```python
from build123d import *

# Parameters (mm, degrees)
F2_W           = 40
F2_H           = 40
F3_DEPTH       = 500
F4_R           = 3
F5_T           = -2
F7_DEPTH       = 40.001
F9_D           = 3.5
F9_CSINK_D     = 6
F9_CSINK_ANGLE = 90


with BuildPart() as f3:
    # F2 (on Front) → F3 (new body, symmetric)
    with BuildSketch(Plane.XZ):
        Rectangle(F2_W, F2_H)
    extrude(amount=F3_DEPTH, both=True)

    # F4
    f4_edges = [f3.edges().sort_by_distance(p)[0] for p in [
        (20, 0, 20),
        (-20, 0, 20),
        (20, 0, -20),
        (-20, 0, -20),
    ]]
    fillet(f4_edges, radius=F4_R)

    # F5
    f5_openings = [f3.faces().sort_by_distance(p)[0] for p in [
        (0, -500, 0),
        (0, 500, 0),
    ]]
    offset(amount=F5_T, openings=f5_openings)

    # F6 (on face) → F7 (cut, through all)
    with BuildSketch(Plane.XY.offset(20)):
        Polygon((20, 500), (-20, 500), (-20, 460), align=None)
        Polygon((20, -500), (-20, -460), (-20, -500), align=None)
    extrude(amount=-F7_DEPTH, mode=Mode.SUBTRACT)

    # F9 (through all)
    with Locations(Plane(origin=(0, 0, -20), x_dir=(1, 0, 0), z_dir=(0, 0, -1))):
        with Locations((0, 360), (0, 120), (0, -120), (0, -360)):
            CounterSinkHole(F9_D / 2, F9_CSINK_D / 2, counter_sink_angle=F9_CSINK_ANGLE)


solid = f3.part
```
The listing builds one solid part. Answer for the finished solid, in the listing's coordinates (mm). A direction names the side the tool comes from. Round coordinates to 2 decimals unless told otherwise and drop trailing zeros. Loops run counter-clockwise (first coordinate to the right, second up) from the corner with the lowest first, then second, coordinate; pieces in that order, holes last.
Q1. Find the intervals of material crossed by line 1 (Z direction, x = -7, y = -291); line 2 (Y direction, x = 0, z = 18.85), in increasing order.
Q2. For a pull along Z with two mould halves and no side action, classify faces 1 (the face through (20, -7, 0)), 2 (the face through (18, -7, 0)), 3 (the face through (0, -7, -20)), 4 (the face through (0, -7, 20)) as released by +Z, released by -Z, zero draft, split by the parting line, or undercut.
Q3. Section A-A, the plane z = -4.5 is taken. Determine the outline of the cut face in (x, y).
Q4. Section B-B, the plane y = 17.5 is taken. Determine the outline of the cut face in (x, z).
Q5. Which of the six approach directions +Z, -Z, +X, -X, +Y, -Y give full straight-line access (tool end or side, diameter ignored) to faces 5 (the face through (0, 480, 19)), 6 (the face through (0, -7, 18))?
Q6. Given pin 1 Ø4.5 at (x, y) = (0, -360) entering from +Z; pin 2 Ø2 at (x, y) = (0, -120) entering from +Z; pin 3 Ø8 at (x, z) = (-15, 10.5) entering from -Y; pin 4 Ø4 at (x, y) = (0, -120) entering from -Z, each flat-ended and moving along its own axis, determine where each tip first touches the part or whether it passes through.
Completed:
1. line 1: z = -20 to -18, 18 to 20
1. line 2: y = -480 to -361.75, -358.25 to -121.75, -118.25 to 118.25, 121.75 to 358.25, 361.75 to 480
2. face 1: zero draft
2. face 2: undercut
2. face 3: released by -Z
2. face 4: released by +Z
3. outline: (-20, -460) - (-18, -462) - (-18, 462) - (-20, 460) - close; (18, -498) - (20, -500) - (20, 500) - (18, 498) - close
4. outline: (-20, -17) arc R3 ccw to (-17, -20) - (17, -20) arc R3 ccw to (20, -17) - (20, 17) arc R3 ccw to (17, 20) - (-17, 20) arc R3 ccw to (-20, 17) - close; hole (-18, -17) arc R1 ccw to (-17, -18) - (17, -18) arc R1 ccw to (18, -17) - (18, 17) arc R1 ccw to (17, 18) - (-17, 18) arc R1 ccw to (-18, 17) - close
5. face 5: +Z, -Z, -X, +Y
5. face 6: +Y, -Y
6. pin 1: stops at z = 20
6. pin 2: passes through
6. pin 3: stops at y = -462
6. pin 4: stops at z = -19
